Autodesk Inventor part; units mm, degrees
ref_plane "YZ Plane" through (0, 0, 0) normal (1, 0, 0) x (0, 1, 0)
ref_plane "XZ Plane" through (0, 0, 0) normal (0, 1, 0) x (-1, 0, 0)
ref_plane "XY Plane" through (0, 0, 0) normal (0, 0, 1) x (1, 0, 0)
sketch "Sketch1" plane through (0, 0, 0) normal (1, 0, 0) x (0, 1, 0)
  line L0 (-62.5, 10) -> (62.5, 10)
  line L1 (62.5, 10) -> (62.5, -10)
  line L2 (62.5, -10) -> (-62.5, -10)
  line L3 (-62.5, -10) -> (-62.5, 10)
  line L4 (-62.5, 10) -> (62.5, -10) construction
  line L5 (62.5, 10) -> (-62.5, -10) construction
  line L6 (60.5, -8) -> (60.5, 8)
  line L7 (60.5, 8) -> (-60.5, 8)
  line L8 (-60.5, 8) -> (-60.5, -8)
  line L9 (-60.5, -8) -> (60.5, -8)
  point P0 (0, 0)
  dimension "d0" = 125
  dimension "d1" = 20
  dimension "d2" = 2
extrude "Extrusion1" add sketch "Sketch1" along normal blind 100
properties part number "Motor Mount" material "Aluminum 6061"
Can you work these out from the model? Positions are in its coordinate system, mm. A direction names the side the tool comes from. Coordinates: 2 decimals unless noted, no trailing zeros. Write each loop counter-clockwise with the first axis right and the second up, starting at its lowest first coordinate (ties: lowest second). Pieces come first, ordered by that corner, then holes. Notation, with made-up numbers: M -3,50.5 L 31,50.5 A11 ccw 31,54.5 Z; hole C 0.25,-16 d6. An arc over 180 degrees is marked long. Write item = value, one per line. Start each with the question number.
Q1. If we section it at C-C, the plane y = 6: Write out the boundary of the cut face in (x, z).
Q2. If I drill on L1, parallel to Y at x = 65.5, z = -3.75; L2, parallel to Z at x = 36.5, y = 47, over which ranges is the centre line in solid material (lowest first)? Write a range as [from, to].
Q3. Thinking about a two-plate mould opening in Z: for faces 1 (the face through (49, -1, 10)), 2 (the face through (49, -62.5, 0)), 3 (the face through (49, 1, 8)), which applies, released by +Z, released by -Z, zero draft, split by the parting line, or undercut?
Q4. If we section it at B-B, the plane x = 90: Write out the boundary of the cut face in (y, z).
Q5. I'm going to push a flat-ended pin straight in: pin 1 (8 mm diameter, centred on y = 29, z = 1, fed in from -X). Where does the tip first touch, or does it pass through?
Q6. If we section it at A-A, the plane z = -1.5: Write out the boundary of the cut face in (x, y), then the cut area to 3 significant figures.
Q7. On a 3-axis mill with a long thin cutter (end or side, diameter ignored), from which of +Z, -Z, +X, -X, +Y, -Y can I reach the whole of each face in a straight line? I mean faces 4 (the face through (49, 60.5, 0)), 5 (the face through (49, 1, -10)). Say none if no direction works.
Check sheet entries:
q1.outline = M 0,-10 L 100,-10 L 100,-8 L 0,-8 Z; M 0,8 L 100,8 L 100,10 L 0,10 Z
q2.L1 = [-62.5, -60.5], [60.5, 62.5]
q2.L2 = [-10, -8], [8, 10]
q3.face_1 = released by +Z
q3.face_2 = zero draft
q3.face_3 = undercut
q4.outline = M -62.5,-10 L 62.5,-10 L 62.5,10 L -62.5,10 Z; hole M -60.5,-8 L 60.5,-8 L 60.5,8 L -60.5,8 Z
q5.pin_1 = through
q6.outline = M 0,-62.5 L 100,-62.5 L 100,-60.5 L 0,-60.5 Z; M 0,60.5 L 100,60.5 L 100,62.5 L 0,62.5 Z
q6.area = 400 mm²
q7.face_4 = +X, -X
q7.face_5 = -Z, +X, -X, +Y, -Y
